```python
from build123d import *

# Parameters (mm, degrees)
F0_W        = 56
F0_H        = 12
F0_W_2      = 52
F0_H_2      = 8
F1_DEPTH    = 90
F1_FACE_W   = 56
F1_FACE_H   = 12
F1_FACE_W_2 = 52
F1_FACE_H_2 = 8
F2_DEPTH    = 2


with BuildPart() as f1:
    # F0 (on Top) → F1 (new body)
    with BuildSketch(Plane.XY):
        with Locations((-19.410297, 19.352412)):
            Rectangle(F0_W, F0_H)
        with Locations((-19.410297, 19.352412)):
            Rectangle(F0_W_2, F0_H_2, mode=Mode.SUBTRACT)
    extrude(amount=F1_DEPTH)

    # F1_face (on face) → F2 (join)
    with BuildSketch(Plane(origin=(-19.410297, 19.352412, 90), x_dir=(1, 0, 0), z_dir=(0, 0, 1))):
        Rectangle(F1_FACE_W, F1_FACE_H)
        Rectangle(F1_FACE_W_2, F1_FACE_H_2, mode=Mode.SUBTRACT)
    extrude(amount=F2_DEPTH)


solid = f1.part
```
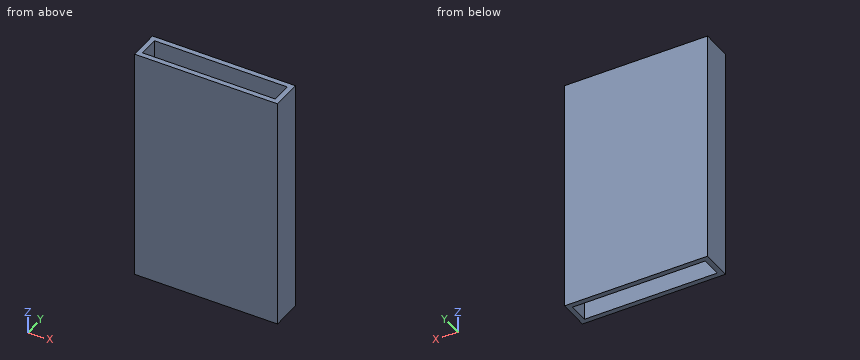
Can you work these out from the model? Positions are in its coordinate system, mm. Coordinates: 2 decimals unless noted, no trailing zeros. Write each loop counter-clockwise with the first axis right and the second up, starting at its lowest first coordinate (ties: lowest second). Pieces come first, ordered by that corner, then holes. Notation, with made-up numbers: (88.25, -31) - (131.25, -31) arc R36 ccw to (131.25, 7) - close; hole circle Ø11 at (21.5, 89.25). An arc over 180 degrees is marked (long way). Return JSON: item names as keys, results as strings.
Q1. If we section it at B-B (x = -4.5): Please give me the cut outline in (y, z), then the cut area to 3 significant figures.
Computed values:
{"outline": "(13.35, 0) - (15.35, 0) - (15.35, 92) - (13.35, 92) - close; (23.35, 0) - (25.35, 0) - (25.35, 92) - (23.35, 92) - close", "area": "368 mm2"}
Q2. If we section it at A-A (y = 16.5): Please give me the cut outline in (x, z).
Computed values:
{"outline": "(-47.41, 0) - (-45.41, 0) - (-45.41, 92) - (-47.41, 92) - close; (6.59, 0) - (8.59, 0) - (8.59, 92) - (6.59, 92) - close"}
Q3. I'm going to push flat-ended pins straight in: pin 1 Ø3 at (x, y) = (-38, 18.5) entering from -Z; pin 2 Ø3 at (x, y) = (-1.5, 15) entering from -Z. Where does each tip first touch, or does it pass through?
Computed values:
{"pin 1": "passes through", "pin 2": "stops at z = 0"}
Q4. If we section it at C-C (z = 17): Please give me the cut outline in (x, y).
Computed values:
{"outline": "(-47.41, 13.35) - (8.59, 13.35) - (8.59, 25.35) - (-47.41, 25.35) - close; hole (-45.41, 15.35) - (6.59, 15.35) - (6.59, 23.35) - (-45.41, 23.35) - close"}
Q5. Please list where these lines run through material, in increasing order: L1, parallel to Y at x = 3.5, z = 77; L2, parallel to X at y = 22.5, z = 75.5. Write a range as from..to.
Computed values:
{"L1": "y = 13.35..15.35, 23.35..25.35", "L2": "x = -47.41..-45.41, 6.59..8.59"}
